```python
from build123d import *

# Parameters (mm, degrees)
EXTRUDE_1_DEPTH     = 1
SKETCH_3_W          = 2.5
SKETCH_3_H          = 2
EXTRUDE_2_DEPTH     = 2.5
CUT_EXTRUDE_1_DEPTH = 2
EXTRUDE_3_DEPTH     = 27.8
SKETCH_5_R          = 1.1
CUT_EXTRUDE_2_DEPTH = 20.3
CUT_EXTRUDE_3_DEPTH = 1.6


with BuildPart() as part:
    # 草图1 → 凸台-拉伸1 (new body)
    with BuildSketch(Plane.XY):
        with BuildLine():
            Line((-9.2, -10.5), (9.2, -10.5))
            ThreePointArc((9.2, -10.5), (10.119238816, -10.119238816), (10.5, -9.2))
            Line((10.5, -9.2), (10.5, 9.2))
            ThreePointArc((10.5, 9.2), (10.119238816, 10.119238816), (9.2, 10.5))
            Line((9.2, 10.5), (-9.2, 10.5))
            ThreePointArc((-9.2, 10.5), (-10.119238816, 10.119238816), (-10.5, 9.2))
            Line((-10.5, 9.2), (-10.5, -9.2))
            ThreePointArc((-10.5, -9.2), (-10.119238816, -10.119238816), (-9.2, -10.5))
        make_face()
    extrude(amount=EXTRUDE_1_DEPTH)

    # 草图3 → 凸台-拉伸2 (add)
    with BuildSketch(Plane.XY.offset(1)):
        with Locations((7.7, -4.2)):
            Rectangle(SKETCH_3_W, SKETCH_3_H)
        with Locations((-7.7, -4.2)):
            Rectangle(SKETCH_3_W, SKETCH_3_H)
        with BuildLine():
            Line((-8.95, -7), (8.95, -7))
            Line((8.95, -7), (8.95, -8.05))
            ThreePointArc((8.95, -8.05), (8.569238816, -8.969238816), (7.65, -9.35))
            Line((7.65, -9.35), (-7.65, -9.35))
            ThreePointArc((-7.65, -9.35), (-8.569238816, -8.969238816), (-8.95, -8.05))
            Line((-8.95, -8.05), (-8.95, -7))
        make_face()
    extrude(amount=EXTRUDE_2_DEPTH)

    # 草图2 → 切除-拉伸1 (cut, through all)
    with BuildSketch(Plane.XY.offset(1)):
        with BuildLine():
            Line((-2.89, -2.15), (2.89, -2.15))
            ThreePointArc((2.89, -2.15), (4.465, -3.725), (2.89, -5.3))
            Line((2.89, -5.3), (-2.89, -5.3))
            ThreePointArc((-2.89, -5.3), (-4.465, -3.725), (-2.89, -2.15))
        make_face()
    extrude(amount=-CUT_EXTRUDE_1_DEPTH, mode=Mode.SUBTRACT)

    # 草图4 → 凸台-拉伸3 (add)
    with BuildSketch(Plane.XY.offset(1)):
        with BuildLine():
            Line((-7.65, 8.8), (7.65, 8.8))
            ThreePointArc((7.65, 8.8), (8.569238816, 8.419238816), (8.95, 7.5))
            Line((8.95, 7.5), (8.95, 5.3))
            Line((8.95, 5.3), (-8.95, 5.3))
            Line((-8.95, 5.3), (-8.95, 7.5))
            ThreePointArc((-8.95, 7.5), (-8.569238816, 8.419238816), (-7.65, 8.8))
        make_face()
    extrude(amount=EXTRUDE_3_DEPTH)

    # 草图5 → 切除-拉伸2 (cut, through all)
    with BuildSketch(Plane(origin=(0, 8.8, 0), x_dir=(1, 0, 0), z_dir=(0, 1, 0))):
        with Locations((0, -21)):
            Circle(SKETCH_5_R)
    extrude(amount=-CUT_EXTRUDE_2_DEPTH, mode=Mode.SUBTRACT)

    # 草图6 → 切除-拉伸3 (cut)
    with BuildSketch(Plane.XZ.offset(-5.3)):
        Polygon((1.125833025, 22.95), (-1.125833025, 22.95), (-2.25166605, 21), (-1.125833025, 19.05), (1.125833025, 19.05), (2.25166605, 21), align=None)
    extrude(amount=-CUT_EXTRUDE_3_DEPTH, mode=Mode.SUBTRACT)


solid = part.part
```
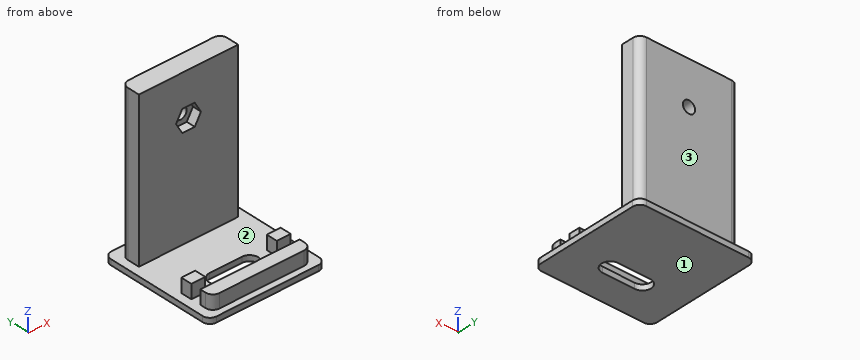
Build history of the part. All positions in model axes, mm. Face numbers are marked on the shaded views. Round coordinates to 2 decimals unless told otherwise and drop trailing zeros. Order: outer loops, then holes, each group sorted by start corner. A loop starts at its lowest first (then second) coordinate and runs counter-clockwise, first axis right, second up. Notation, with made-up numbers: (48.5, 73.5) -> (82.5, 73.5) arc R21 ccw to (82.5, 78.5) -> close; hole circle Ø9 at (80.25, 73.25). An arc over 180 degrees is marked (long way). Answer in a Markdown table with one row per item.
1) Band-saw the part on C-C on y = 0.5. Give the cut face in (x, z), and give its area (3 significant figures).
Values:
| item | result |
|---|---|
| outline | (-10.5, 0) -> (10.5, 0) -> (10.5, 1) -> (-10.5, 1) -> close |
| area | 21.0 mm2 |
2) Band-saw the part on B-B on z = 6.5. Give the cut face in (x, y), and give its area (3 significant figures).
Values:
| item | result |
|---|---|
| outline | (-8.95, 5.3) -> (8.95, 5.3) -> (8.95, 7.5) arc R1.3 ccw to (7.65, 8.8) -> (-7.65, 8.8) arc R1.3 ccw to (-8.95, 7.5) -> close |
| area | 61.9 mm2 |
3) Mould opens along Y. For the marked faces 1, 2 and 3 say: released by +Y, released by -Y, zero draft, split by the parting line, or undercut.
Values:
| item | result |
|---|---|
| face 1 | zero draft |
| face 2 | undercut |
| face 3 | released by +Y |
4) Band-saw the part on A-A on x = 0. Give the cut face in (y, z), and give its area (3 significant figures).
Values:
| item | result |
|---|---|
| outline | (-10.5, 0) -> (-5.3, 0) -> (-5.3, 1) -> (-7, 1) -> (-7, 3.5) -> (-9.35, 3.5) -> (-9.35, 1) -> (-10.5, 1) -> close; (-2.15, 0) -> (10.5, 0) -> (10.5, 1) -> (8.8, 1) -> (8.8, 19.9) -> (6.9, 19.9) -> (6.9, 19.05) -> (5.3, 19.05) -> (5.3, 1) -> (-2.15, 1) -> close; (5.3, 22.95) -> (6.9, 22.95) -> (6.9, 22.1) -> (8.8, 22.1) -> (8.8, 28.8) -> (5.3, 28.8) -> close |
| area | 111 mm2 |
5) Wall check: L1, parallel to Y at x = -7, z = 1.25; L2, parallel to X at y = 7.55, z = 21; L3, parallel to Z at x = 0, y = 7.95. Give the ranges that are in metal, low to high.
Values:
| item | result |
|---|---|
| L1 | -9.35 to -7, -5.2 to -3.2, 5.3 to 8.8 |
| L2 | -8.95 to -1.1, 1.1 to 8.95 |
| L3 | 0 to 19.9, 22.1 to 28.8 |
6) Pin check, flat tips, straight feed: P1, Ø0.7, axis at x = 8.5, z = 1.5, coming from the -Y side; P2, Ø3.5, axis at x = 0, z = 21, coming from the +Y side; P3, Ø0.6, axis at x = -8, y = -4, coming from the +Z side. Stop position of each tip, or through.
Values:
| item | result |
|---|---|
| P1 | y = -9.25 |
| P2 | y = 8.8 |
| P3 | z = 3.5 |
